Verification items for the finished model (mm, model axes). A direction names the side the tool comes from. Give positions to 0.01 mm unless a question says otherwise; leave off trailing zeros. Write each loop counter-clockwise with the first axis right and the second up, starting at its lowest first coordinate (ties: lowest second). Pieces come first, ordered by that corner, then holes.
Autodesk Inventor part; units mm, degrees
ref_plane "YZ Plane" through (0, 0, 0) normal (1, 0, 0) x (0, 1, 0)
ref_plane "XZ Plane" through (0, 0, 0) normal (0, 1, 0) x (-1, 0, 0)
ref_plane "XY Plane" through (0, 0, 0) normal (0, 0, 1) x (1, 0, 0)
sketch "Sketch1" plane through (0, 0, 0) normal (0, 0, 1) x (1, 0, 0)
  line L0 (-3.5, -5) -> (3.5, -5)
  line L1 (3.5, -5) -> (3.5, 5)
  line L2 (3.5, 5) -> (-3.5, 5)
  line L3 (-3.5, 5) -> (-3.5, -5)
  line L4 (-3.5, -5) -> (3.5, 5) construction
  line L5 (3.5, -5) -> (-3.5, 5) construction
  point P0 (0, 0)
  dimension "d0" = 7
  dimension "d1" = 10
extrude "Extrusion1" add sketch "Sketch1" along normal blind 300
sketch "Sketch2" plane through (3.5, -5, 0) normal (1, 0, 0) x (0, 0, -1)
  point P0 (0, 5)
sketch "Sketch3" plane through (3.5, -5, 0) normal (1, 0, 0) x (0, 0, -1)
  line L0 (0, 10) -> (-300, 10)
  line L1 (0, 0) -> (-300, 0)
  line L2 (-275, 10) -> (-280, 10)
  line L3 (-280, 10) -> (-280, 0)
  line L4 (-280, 0) -> (-275, 0)
  line L5 (-275, 0) -> (-275, 10)
  line L6 (-300, 0) -> (-300, 10)
  point P0 (0, 5)
  point P1 (-275, 0)
  point P2 (-280, 10)
  dimension "d4" = 5
  dimension "d12" = 20
extrude "Extrusion2" add sketch "Sketch3" along normal blind 85.85 contours L5 L1 L3 L0
sketch "Sketch4" plane through (-3.5, 5, 300) normal (0, 1, 0) x (1, 0, 0)
  circle A0 centre (87.8562, 22.5) radius 1.64
  line L0 (7, 25) -> (92.85, 25)
  point P0 (3.5, 300)
  dimension "d7" = 3.28
  dimension "d8" = 2.5
extrude "Extrusion3" cut sketch "Sketch4" against normal through all
fillet "Fillet1" radius 2 2 edges at (89.35, 0, 275) (89.35, 0, 280)
properties part number "support_rod_left"
Item 1: Depth check by flat-ended pin: pin 1 (1.5 mm diameter, centred on x = 16, y = -1.5, fed in from +Z); pin 2 (4 mm diameter, centred on x = 77.5, y = 2.5, fed in from -Z); pin 3 (3 mm diameter, centred on y = -0.5, z = 196, fed in from +X); pin 4 (3 mm diameter, centred on x = 84.36, z = 277.5, fed in from +Y). Enter the tip coordinate at first touch or a pass-through.
Answer key:
pin 1: stops at z = 280
pin 2: stops at z = 275
pin 3: stops at x = 3.5
pin 4: passes through
Item 2: Sectioned sample at C-C on x = 22. Record the cut outline in (y, z), then the cut area to 3 significant figures.
Answer key:
outline: (-5, 275) - (5, 275) - (5, 280) - (-5, 280) - close
area: 50.0 mm2
Item 3: Scan lines: line 1 along X through (y, z) = (0.75, 277.5); line 2 along X through (y, z) = (-3.75, 58.5); line 3 along Z through (x, y) = (29, 1.5). Record each from-to range of solid material in increasing order.
Answer key:
line 1: x = -3.5 to 82.72, 86 to 89.35
line 2: x = -3.5 to 3.5
line 3: z = 275 to 280
Item 4: Sectioned sample at A-A on y = -0.25. Record the cut outline in (x, z).
Answer key:
outline: (-3.5, 0) - (3.5, 0) - (3.5, 275) - (87.35, 275) arc R2 ccw to (89.35, 277) - (89.35, 278) arc R2 ccw to (87.35, 280) - (3.5, 280) - (3.5, 300) - (-3.5, 300) - close; hole circle Ø3.28 at (84.36, 277.5)
Item 5: Sectioned sample at B-B on z = 206. Record the cut outline in (x, y), then the cut area to 3 significant figures.
Answer key:
outline: (-3.5, -5) - (3.5, -5) - (3.5, 5) - (-3.5, 5) - close
area: 70.0 mm2
Item 6: Set-up check for faces 1 (the face through (3.5, 0, 290)), 2 (the face through (-3.5, 0, 148)), 3 (the face through (3.5, 0, 136)): record each of +Z, -Z, +X, -X, +Y, -Y from which the full face is reachable in a straight line by a thin tool's end or side.
Answer key:
face 1: +Z, +X, +Y, -Y
face 2: +Z, -Z, -X, +Y, -Y
face 3: -Z, +X, +Y, -Y
